The model under review builds one solid part; all positions refer to its coordinate system, in mm. Coordinates: 2 decimals unless noted, no trailing zeros. Order: outer loops, then holes, each group sorted by start corner. A loop starts at its lowest first (then second) coordinate and runs counter-clockwise, first axis right, second up. Notation, with made-up numbers: (79, 66) - (96, 66) arc R27 ccw to (96, 102) - close; hole circle Ø11 at (59, 52.25). An arc over 180 degrees is marked (long way). Answer in a Markdown table with one row per item.
```python
from build123d import *

# Parameters (mm, degrees)
F0_W     = 3.9624
F0_H     = 3.9624
F1_DEPTH = 339.725
F2_W     = 3.9624
F2_H     = 3.9624
F3_DEPTH = 6.35
F4_R     = 1.98119


# Not quite as in the source:
# - a fillet or chamfer is up to 0.001 mm smaller than in the source, because OpenCascade refuses the exact size


with BuildPart() as f1:
    # F0 (on Front) → F1 (new body)
    with BuildSketch(Plane.XZ):
        Rectangle(F0_W, F0_H)
    extrude(amount=F1_DEPTH)

    # F2 (on face) → F3 (join)
    with BuildSketch(Plane.YZ.offset(1.9812)):
        with Locations((-337.7438, 0)):
            Rectangle(F2_W, F2_H)
        with Locations((-1.9812, 0)):
            Rectangle(F2_W, F2_H)
    extrude(amount=F3_DEPTH)

    # F4 (radius 1.9812 in the source; OpenCascade refuses exactly that, so slightly less here)
    f4_edges = [f1.edges().sort_by_distance(p)[0] for p in [
        (3.175, 0, 1.9812),
        (3.175, 0, -1.9812),
        (-1.9812, -169.8625, 1.9812),
        (1.9812, -169.8625, 1.9812),
        (-1.9812, -169.8625, -1.9812),
        (1.9812, -169.8625, -1.9812),
        (-1.9812, 0, 0),
        (3.175, -339.725, 1.9812),
        (3.175, -339.725, -1.9812),
        (-1.9812, -339.725, 0),
        (5.1562, -335.7626, -1.9812),
        (5.1562, -3.9624, -1.9812),
        (5.1562, -335.7626, 1.9812),
        (5.1562, -3.9624, 1.9812),
    ]]
    fillet(f4_edges, radius=F4_R)


solid = f1.part
```
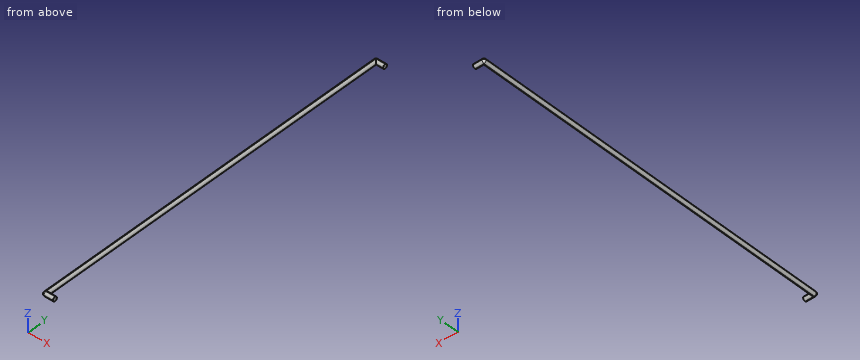
Item 1: To check wall thickness, follow line 1 (Y direction, x = 3.5, z = 0.25); line 2 (Y direction, x = 0.75, z = -0.2); line 3 (Y direction, x = 4, z = 0.65). State the ranges of each line that lie inside material, in increasing order. Write a range as from..to.
Check values:
| item | result |
|---|---|
| line 1 | -339.71..-335.78, -3.95..-0.02 |
| line 2 | -339.71..-0.01 |
| line 3 | -339.62..-335.87, -3.85..-0.11 |
Item 2: Clearance check with flat-ended pins moving along their axes: pin 1 Ø1 at (x, z) = (5, -0.5) entering from -Y (3 decimals); pin 2 Ø1 at (y, z) = (-304, 0.5) entering from +X; pin 3 Ø1 at (y, z) = (-220, -1.5) entering from -X. State where each tip first meets the part, or that it passes through.
Check values:
| item | result |
|---|---|
| pin 1 | y = -339.725 |
| pin 2 | x = 1.98 |
| pin 3 | x = -1.71 |
Item 3: We need section C-C, the plane z = 0.65. Write out the cut boundary in (x, y), then the cut area to 3 significant figures.
Check values:
| item | result |
|---|---|
| outline | (-1.87, -337.74) arc R1.87 ccw to (0, -339.62) - (8.33, -339.62) - (8.33, -335.87) - (1.87, -335.87) - (1.87, -3.85) - (8.33, -3.85) - (8.33, -0.11) - (0, -0.11) arc R1.87 ccw to (-1.87, -1.98) - close |
| area | 1,320 mm^2 |
